from build123d import *

# Parameters (mm, degrees)
EXTRUDE_1_DEPTH      = 10
EXTRUDE_2_DEPTH      = 5
EXTRUDE_2_DEPTH_BACK = 5
SKETCH_3_W           = 29
SKETCH_3_H           = 50
CUT_EXTRUDE_2_DEPTH  = 5


with BuildPart() as part:
    # 스케치1 → 보스-돌출1 (new body)
    with BuildSketch(Plane(origin=(0, 0, 0), x_dir=(1, 0, 0), z_dir=(0, 1, 0))):
        Polygon((-14.5, 0), (-8, 0), (-8, 19), (8, 19), (8, 0), (14.5, 0), (14.5, 25), (-14.5, 25), align=None)
    extrude(amount=EXTRUDE_1_DEPTH)

    # 스케치2 → 보스-돌출2 (add, two sides)
    with BuildSketch(Plane(origin=(0, 10, 0), x_dir=(1, 0, 0), z_dir=(0, 1, 0))) as extrude_2_sk:
        Polygon((-8, 0), (-19.5, 0), (-19.5, 30), (19.5, 30), (19.5, 0), (8, 0), (8, 19), (-8, 19), align=None)
    extrude(amount=EXTRUDE_2_DEPTH)
    extrude(extrude_2_sk.sketch, amount=-EXTRUDE_2_DEPTH_BACK)

    # 스케치3 → 컷-돌출2 (cut)
    with BuildSketch(Plane(origin=(0, 15, 0), x_dir=(1, 0, 0), z_dir=(0, 1, 0))):
        Rectangle(SKETCH_3_W, SKETCH_3_H)
    extrude(amount=-CUT_EXTRUDE_2_DEPTH, mode=Mode.SUBTRACT)


solid = part.part
Model file for the job. Use its own axes, mm. A direction names the side the tool comes from. Give positions to 0.01 mm unless a question says otherwise; leave off trailing zeros. Order: outer loops, then holes, each group sorted by start corner. A loop starts at its lowest first (then second) coordinate and runs counter-clockwise, first axis right, second up. Notation, with made-up numbers: (-23.75, 10.25) - (33.25, 10.25) arc R14 cw to (33.25, 28.25) - close; hole circle Ø6 at (84, 84.25). An arc over 180 degrees is marked (long way). One line per item, written item: value.
Item 1: Slice it at B-B (x = -10). List the corners of the cut face in (y, z), then the cut area to 3 significant figures.
Response values:
outline: (0, -25) - (5, -25) - (5, -30) - (15, -30) - (15, -25) - (10, -25) - (10, 0) - (0, 0) - close
area: 300 mm2
Item 2: Slice it at C-C (y = 10.5). List the corners of the cut face in (x, z).
Response values:
outline: (-19.5, -30) - (19.5, -30) - (19.5, 0) - (14.5, 0) - (14.5, -25) - (-14.5, -25) - (-14.5, 0) - (-19.5, 0) - close
Item 3: Tool access for faces 1 (the flat face through (-14.5, 2, -13)), 2 (the flat face through (14.5, 13, -12)), 3 (the flat face through (0, 2, -25)), 4 (the flat face through (14.5, 2, -12)), 5 (the flat face through (0, 5, -19)): list every direction of +Z, -Z, +X, -X, +Y, -Y with a clear straight run to the whole face (end or side of a thin tool).
Response values:
face 1: +Z, -Z, -X, -Y
face 2: +Z, +Y
face 3: -Z, +X, -X, -Y
face 4: +Z, -Z, +X, -Y
face 5: +Z, +Y, -Y
Item 4: Pin check, flat tips, straight feed: pin 1 Ø1.5 at (x, y) = (7, 2) entering from -Z; pin 2 Ø5 at (x, y) = (-2, 4) entering from +Z; pin 3 Ø4 at (x, y) = (-1, 13.5) entering from +Z. Stop position of each tip, or through.
Response values:
pin 1: z = -25
pin 2: z = -19
pin 3: z = -25
Item 5: Wall check: line 1 (X direction, y = 9, z = -3.5); line 2 (X direction, y = 2, z = -4.5); line 3 (Y direction, x = 8, z = -24). Give the ranges that are in metal, low to high.
Response values:
line 1: -19.5 to -8, 8 to 19.5
line 2: -14.5 to -8, 8 to 14.5
line 3: 0 to 10
Item 6: Slice it at A-A (z = -7.75). List the corners of the cut face in (x, y).
Response values:
outline: (-19.5, 5) - (-14.5, 5) - (-14.5, 0) - (-8, 0) - (-8, 10) - (-14.5, 10) - (-14.5, 15) - (-19.5, 15) - close; (8, 0) - (14.5, 0) - (14.5, 5) - (19.5, 5) - (19.5, 15) - (14.5, 15) - (14.5, 10) - (8, 10) - close
Item 7: Slice it at D-D (z = -24.25). List the corners of the cut face in (x, y), then the cut area to 3 significant figures.
Response values:
outline: (-19.5, 5) - (-14.5, 5) - (-14.5, 0) - (14.5, 0) - (14.5, 5) - (19.5, 5) - (19.5, 15) - (14.5, 15) - (14.5, 10) - (-14.5, 10) - (-14.5, 15) - (-19.5, 15) - close
area: 390 mm2
